Could you check a few things on this model? Use its own coordinates, in mm. Face numbers are marked on the shaded views. Coordinates: 2 decimals unless noted, no trailing zeros. Loops run counter-clockwise (first coordinate to the right, second up) from the corner with the lowest first, then second, coordinate; pieces in that order, holes last. Notation, with made-up numbers: (23, -30) - (70, -30) arc R10 ccw to (70, -22) - close; hole circle Ø2 at (39.25, 61.25). An arc over 180 degrees is marked (long way). One line per item, written item: value. Start each with the question number.
(1) If we section it at A-A on y = 0.5: Write out the boundary of the cut face in (x, z), then the cut area to 3 significant figures.
(2) If we section it at C-C on x = 0: Write out the boundary of the cut face in (y, z).
(3) I'm going to push flat-ended pins straight in: P1, Ø1.6, axis at x = 8.5, z = 0, coming from the -Y side; P2, Ø7.5, axis at x = 0.5, z = 0.5, coming from the -Y side; P3, Ø2.5, axis at x = -9, z = -3.5, coming from the -Y side. Where does each tip first touch, or does it pass through?
(4) If I drill on line 1 along X through (y, z) = (0.1, 0); line 2 along Z through (x, y) = (7.5, 6.25); line 3 along X through (y, z) = (8, 8.5), over which ranges is the centre line in solid material (lowest first)? Write a range as from..to.
(5) If we section it at B-B on y = 3.75: Count the separate pieces of the cut face and the enclosed holes in it, then the cut area to 3 significant figures.
(6) If we mould it in two halves opening along Z, with no side actions, what happens to the marked faces 1, 2 and 3? For each: pulls with the +Z half, pulls with the -Z half, needs draft (parallel to the pull), parting line crosses it, or undercut.
```python
from build123d import *

# Parameters (mm, degrees)
SKETCH1_R           = 3.5
BOSS_EXTRUDE1_DEPTH = 10
SKETCH2_R           = 12.5
BOSS_EXTRUDE2_DEPTH = 1
BOSS_EXTRUDE3_START = 9
SKETCH3_R           = 12.5
SKETCH3_R_2         = 11.5
BOSS_EXTRUDE3_DEPTH = 9
BOSS_EXTRUDE4_START = 12
SKETCH3_4_R         = 12.5
SKETCH3_4_R_2       = 11.5
BOSS_EXTRUDE4_DEPTH = 12
CHAMFER1_SIZE       = 1
CUT_EXTRUDE4_START  = -1
CUT_EXTRUDE4_DEPTH  = 1
CHAMFER2_SIZE       = 0.25


with BuildPart() as part:
    # Sketch1 → Boss-Extrude1 (new body)
    with BuildSketch(Plane(origin=(0, 0, 0), x_dir=(1, 0, 0), z_dir=(0, 1, 0))):
        with Locations(Location((0, 0, 0), (0, 0, 270))):
            Circle(SKETCH1_R)
        with BuildLine():
            Line((-1.75, 1.038612788), (1.75, 1.038612788))
            Line((1.75, 1.038612788), (1.75, 2.738612788))
            ThreePointArc((1.75, 2.738612788), (0, -3.25), (-1.75, 2.738612788))
            Line((-1.75, 2.738612788), (-1.75, 1.038612788))
        make_face(mode=Mode.SUBTRACT)
    extrude(amount=BOSS_EXTRUDE1_DEPTH)

    # Sketch2 → Boss-Extrude2 (add)
    with BuildSketch(Plane(origin=(0, 10, 0), x_dir=(1, 0, 0), z_dir=(0, 1, 0))):
        with Locations(Location((0, 0, 0), (0, 0, 270))):
            Circle(SKETCH2_R)
    extrude(amount=BOSS_EXTRUDE2_DEPTH)

    # Sketch3 → Boss-Extrude3 (add)
    # profile 1 of 8: a face of its own
    with BuildSketch(Plane.XZ.offset(-10).offset(BOSS_EXTRUDE3_START)):
        with Locations(Location((0, 0, 0), (0, 0, 270))):
            Circle(SKETCH3_R)
        Circle(SKETCH3_R_2, mode=Mode.SUBTRACT)
    # profile 2 of 8: a face of its own
    with BuildSketch(Plane.XZ.offset(-10).offset(BOSS_EXTRUDE3_START)):
        with BuildLine():
            Line((-6.594245022, 9.421567416), (-2.543076387, 2.40473751))
            ThreePointArc((-2.543076387, 2.40473751), (-1.75, 3.031088913), (-0.811025579, 3.40473751))
            Line((-0.811025579, 3.40473751), (-4.862194215, 10.421567416))
            ThreePointArc((-4.862194215, 10.421567416), (-5.75, 9.959292144), (-6.594245022, 9.421567416))
        make_face()
    # profile 3 of 8: a face of its own
    with BuildSketch(Plane.XZ.offset(-10).offset(BOSS_EXTRUDE3_START)):
        with BuildLine():
            Line((-11.5, 0), (-3.5, 0))
            ThreePointArc((-3.5, 0), (-3.463333429, 0.505293538), (-3.354101966, 1))
            Line((-3.354101966, 1), (-11.456439237, 1))
            ThreePointArc((-11.456439237, 1), (-11.489104648, 0.50047416), (-11.5, 0))
        make_face()
    # profile 4 of 8: a face of its own
    with BuildSketch(Plane.XZ.offset(-10).offset(BOSS_EXTRUDE3_START)):
        with BuildLine():
            ThreePointArc((-3.354101966, -1), (-3.463333429, -0.505293538), (-3.5, 0))
            Line((-3.5, 0), (-11.5, 0))
            ThreePointArc((-11.5, 0), (-11.489104648, -0.50047416), (-11.456439237, -1))
            Line((-11.456439237, -1), (-3.354101966, -1))
        make_face()
    # profile 5 of 8: a face of its own
    with BuildSketch(Plane.XZ.offset(-10).offset(BOSS_EXTRUDE3_START)):
        with BuildLine():
            Line((11.456439237, 1), (3.354101966, 1))
            ThreePointArc((3.354101966, 1), (3.463333429, 0.505293538), (3.5, 0))
            ThreePointArc((3.5, 0), (3.463333429, -0.505293538), (3.354101966, -1))
            Line((3.354101966, -1), (11.456439237, -1))
            ThreePointArc((11.456439237, -1), (11.489104648, -0.50047416), (11.5, 0))
            ThreePointArc((11.5, 0), (11.489104648, 0.50047416), (11.456439237, 1))
        make_face()
    # profile 6 of 8: a face of its own
    with BuildSketch(Plane.XZ.offset(-10).offset(BOSS_EXTRUDE3_START)):
        with BuildLine():
            ThreePointArc((2.543076387, -2.40473751), (1.75, -3.031088913), (0.811025579, -3.40473751))
            Line((0.811025579, -3.40473751), (4.862194215, -10.421567416))
            ThreePointArc((4.862194215, -10.421567416), (5.75, -9.959292144), (6.594245022, -9.421567416))
            Line((6.594245022, -9.421567416), (2.543076387, -2.40473751))
        make_face()
    # profile 7 of 8: a face of its own
    with BuildSketch(Plane.XZ.offset(-10).offset(BOSS_EXTRUDE3_START)):
        with BuildLine():
            ThreePointArc((-0.811025579, -3.40473751), (-1.75, -3.031088913), (-2.543076387, -2.40473751))
            Line((-2.543076387, -2.40473751), (-6.594245022, -9.421567416))
            ThreePointArc((-6.594245022, -9.421567416), (-5.75, -9.959292144), (-4.862194215, -10.421567416))
            Line((-4.862194215, -10.421567416), (-0.811025579, -3.40473751))
        make_face()
    # profile 8 of 8: a face of its own
    with BuildSketch(Plane.XZ.offset(-10).offset(BOSS_EXTRUDE3_START)):
        with BuildLine():
            Line((4.862194215, 10.421567416), (0.811025579, 3.40473751))
            ThreePointArc((0.811025579, 3.40473751), (1.75, 3.031088913), (2.543076387, 2.40473751))
            Line((2.543076387, 2.40473751), (6.594245022, 9.421567416))
            ThreePointArc((6.594245022, 9.421567416), (5.75, 9.959292144), (4.862194215, 10.421567416))
        make_face()
    extrude(amount=-BOSS_EXTRUDE3_DEPTH)

    # Sketch3<4> → Boss-Extrude4 (add)
    with BuildSketch(Plane.XZ.offset(-10).offset(BOSS_EXTRUDE4_START)):
        with Locations(Location((0, 0, 0), (0, 0, 270))):
            Circle(SKETCH3_4_R)
        with Locations(Location((0, 0, 0), (0, 0, 64.988541976))):
            Circle(SKETCH3_4_R_2, mode=Mode.SUBTRACT)
    extrude(amount=-BOSS_EXTRUDE4_DEPTH)

    # Chamfer1
    chamfer1_edges = [part.edges().sort_by_distance(p)[0] for p in [
        (0, 11, -12.5),
    ]]
    chamfer(chamfer1_edges, length=CHAMFER1_SIZE - 0.0001)  # a hair under: the kernel refuses the full size

    # Sketch4 → Cut-Extrude4 (cut)
    with BuildSketch(Plane(origin=(0, 11, 0), x_dir=(1, 0, 0), z_dir=(0, 1, 0)).offset(CUT_EXTRUDE4_START)):
        with BuildLine():
            Line((6.489125293, 0.5), (6.489125293, 0))
            Line((6.489125293, 0), (11.5, 0))
            ThreePointArc((11.5, 0), (11.497281002, 0.250059123), (11.489125293, 0.5))
            Line((11.489125293, 0.5), (6.489125293, 0.5))
        make_face()
        with BuildLine():
            Line((11.5, 0), (6.489125293, 0))
            Line((6.489125293, 0), (6.489125293, -0.5))
            Line((6.489125293, -0.5), (11.489125293, -0.5))
            ThreePointArc((11.489125293, -0.5), (11.497281002, -0.250059123), (11.5, 0))
        make_face()
    extrude(amount=CUT_EXTRUDE4_DEPTH, mode=Mode.SUBTRACT)

    # Chamfer2
    chamfer2_edges = [part.edges().sort_by_distance(p)[0] for p in [
        (6.489125293, 11, 0),
        (8.989125293, 11, -0.5),
        (8.989125293, 11, 0.5),
    ]]
    chamfer(chamfer2_edges, length=CHAMFER2_SIZE)


solid = part.part
```
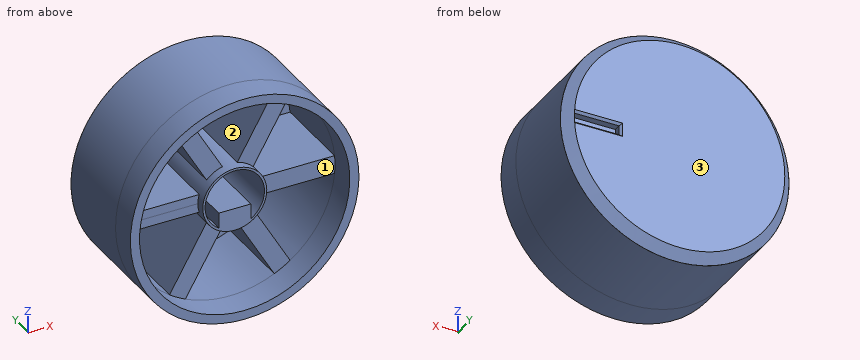
Values:
1. outline: circle Ø25 at (0, 0); circle Ø7 at (0, 0); hole circle Ø23 at (0, 0); hole (-1.75, -2.74) - (-1.75, -1.04) - (1.75, -1.04) - (1.75, -2.74) arc R3.25 ccw (long way) to start
1. area: 87.9 mm2
2. outline: (-2, -12.5) - (10, -12.5) - (11, -11.5) - (11, 11.5) - (10, 12.5) - (-2, 12.5) - (-2, 11.5) - (10, 11.5) - (10, 3.5) - (0, 3.5) - (0, 3.25) - (10, 3.25) - (10, -1.04) - (0, -1.04) - (0, -3.5) - (10, -3.5) - (10, -11.5) - (-2, -11.5) - close
3. P1: stops at y = 1
3. P2: stops at y = 0
3. P3: stops at y = 10
4. line 1: x = -12.5..-11.5, -3.5..-3.25, 3.25..3.5, 11.5..12.5
4. line 2: z = -10..-8.72, -1..1, 8.72..10
4. line 3: x = -9.17..-7.75, -6.06..-3.75, 3.75..6.06, 7.75..9.17
5. separate pieces: 1
5. enclosed holes: 7
5. area: 184 mm2
6. face 1: undercut
6. face 2: undercut
6. face 3: needs draft
